Could you check a few things on this model? Use its own coordinates, in mm. Face numbers are marked on the shaded views. Give positions to 0.01 mm unless a question says otherwise; leave off trailing zeros. Loops run counter-clockwise (first coordinate to the right, second up) from the corner with the lowest first, then second, coordinate; pieces in that order, holes last. Notation, with made-up numbers: M 65.5,-13.5 L 121.5,-13.5 A30 cw 121.5,24.5 Z; hole C 48,57 d6. An arc over 180 degrees is marked long. Return JSON: item names as keys, results as strings. Group by question number.
1. If we mould it in two halves opening along Y, with no side actions, what happens to the marked faces 1, 2, 3 and 4? For each: +Y half, -Y half, draft (parallel to the pull), parting line (faces both ways), or undercut.
2. Please list where these lines run through material, in increasing order: line 1 (Y direction, x = 0, z = -38); line 2 (Y direction, x = -16.5, z = -24.5); line 3 (X direction, y = 12, z = -21).
3. If we section it at A-A (z = -22.5): Write out the boundary of the cut face in (x, y), plus the area to 3 significant figures.
4. For pin 1 (5 mm diameter, centred on x = 1, z = -28.5, fed in from -Y); pin 2 (8 mm diameter, centred on x = 24.5, z = -29.5, fed in from +Y), each with a flat end and sliding along its axis, tell me the tip position at first contact or that it passes through.
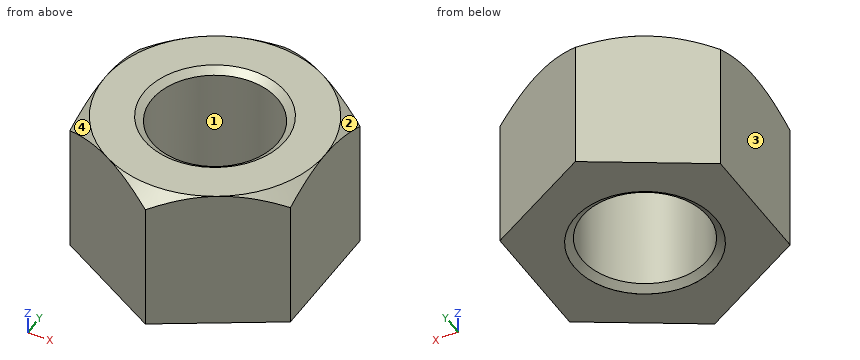
```python
from build123d import *

# Parameters (mm, degrees)
THREADSCHEMATIC_START     = -51.9176
THREADSCHEMATIC_OUTLINE_R = 22.62124
THREADSCHEMATIC_DEPTH     = 51.9176


# Read off the part's stored shape, not the designer's step: ThreadSchematic
with BuildPart() as part:
    # ThreadSchematic outline → ThreadSchematic (new body)
    with BuildSketch(Plane.XY.offset(THREADSCHEMATIC_START)):
        Polygon((39.6875, 22.913588808), (0, 45.827177617), (-39.6875, 22.913588808), (-39.6875, -22.913588808), (0, -45.827177617), (39.6875, -22.913588808), align=None)
        Circle(THREADSCHEMATIC_OUTLINE_R, mode=Mode.SUBTRACT)
    extrude(amount=THREADSCHEMATIC_DEPTH)

    # Sketch2 → Single-Chamfer (revolve, cut)
    with BuildSketch(Plane(origin=(0, 0, 0), x_dir=(0, 0, -1), z_dir=(1, 0, 0))):
        Polygon((0, 39.6875), (-12.7, 39.6875), (-12.7, 58.527177617), (5.08, 58.527177617), (5.08, 45.827177617), align=None)
    revolve(axis=Axis((0, 0, 0), (0, 0, -1)), mode=Mode.SUBTRACT)

    # Sketch3 → EndChamfer (revolve, cut)
    with BuildSketch(Plane(origin=(0, 0, 0), x_dir=(0, 0, -1), z_dir=(1, 0, 0)), mode=Mode.PRIVATE) as endchamfer_sk:
        Polygon((51.8922, 25.4), (49.751920431, 22.343364), (51.943, 22.343364), (51.943, 25.4), align=None)
        Polygon((-0.0508, 25.4), (0, 25.4), (2.140279569, 22.343364), (-0.0508, 22.343364), align=None)
    revolve(endchamfer_sk.sketch.rotate(Axis((0, 0, -25.037505729), (0, 0, -1)), 90), axis=Axis((0, 0, -25.037505729), (0, 0, -1)), mode=Mode.SUBTRACT)


solid = part.part
```
Answer:
{
 "1": {"face 1": "undercut", "face 2": "+Y half", "face 3": "draft", "face 4": "-Y half"},
 "2": {"line 1": "y = -45.83 to -22.62, 22.62 to 45.83", "line 2": "y = -36.3 to -15.47, 15.47 to 36.3", "line 3": "x = -39.69 to -19.18, 19.18 to 39.69"},
 "3": {"outline": "M -39.69,-22.91 L 0,-45.83 L 39.69,-22.91 L 39.69,22.91 L 0,45.83 L -39.69,22.91 Z; hole C 0,0 d45.24", "area": "3,850 mm²"},
 "4": {"pin 1": "stops at y = -45.83", "pin 2": "stops at y = 33.99"}
}
